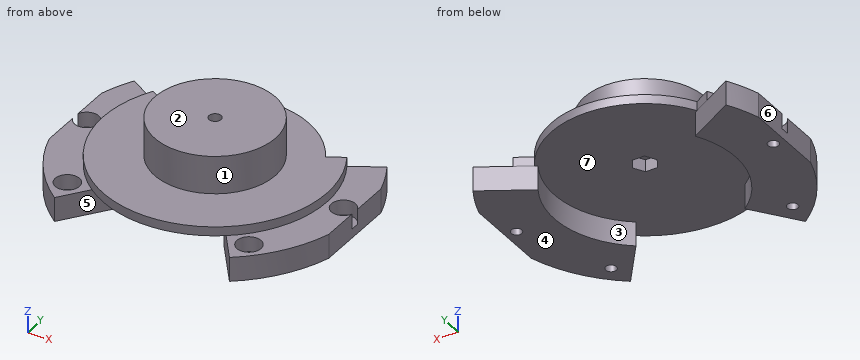
from build123d import *

# Parameters (mm, degrees)
SKETCH1_R           = 48.25
BOSS_EXTRUDE1_DEPTH = 8
SKETCH2_W           = 17.162038191
SKETCH2_H           = 56.822210482
SKETCH2_W_2         = 16.152506533
SKETCH2_H_2         = 65.186901365
CUT_EXTRUDE1_DEPTH  = 8
SKETCH3_R           = 30
CUT_EXTRUDE2_DEPTH  = 8
SKETCH4_R           = 1.75
CUT_EXTRUDE3_DEPTH  = 10
CIRPATTERN1_COUNT   = 8
CUT_EXTRUDE4_DEPTH  = 10
CIRPATTERN2_COUNT   = 2
SKETCH9_R           = 4
CUT_EXTRUDE5_DEPTH  = 5
CIRPATTERN3_COUNT   = 8
SKETCH10_R          = 4
CUT_EXTRUDE6_DEPTH  = 5
SKETCH11_R          = 37
BOSS_EXTRUDE2_DEPTH = 3
SKETCH12_R          = 20
BOSS_EXTRUDE3_DEPTH = 12.5
SKETCH13_R          = 2
CUT_EXTRUDE8_DEPTH  = 38
CUT_EXTRUDE9_DEPTH  = 4
CUT_EXTRUDE10_DEPTH = 10
CUT_EXTRUDE11_START = 14
CUT_EXTRUDE11_DEPTH = 14


with BuildPart() as part:
    # Sketch1 → Boss-Extrude1 (new body)
    with BuildSketch(Plane.XY):
        Circle(SKETCH1_R)
    extrude(amount=-BOSS_EXTRUDE1_DEPTH)

    # Sketch2 → Cut-Extrude1 (cut)
    with BuildSketch(Plane.XY):
        with Locations((-54.831019095, 0)):
            Rectangle(SKETCH2_W, SKETCH2_H)
        with Locations((54.326253267, -4.182345442)):
            Rectangle(SKETCH2_W_2, SKETCH2_H_2)
    extrude(amount=-CUT_EXTRUDE1_DEPTH, mode=Mode.SUBTRACT)

    # Sketch3 → Cut-Extrude2 (cut)
    with BuildSketch(Plane.XY):
        Circle(SKETCH3_R)
    extrude(amount=-CUT_EXTRUDE2_DEPTH, mode=Mode.SUBTRACT)

    # Sketch4 → Cut-Extrude3 (cut)
    with BuildSketch(Plane.XY):
        with Locations((-42.5, 0)):
            Circle(SKETCH4_R)
    cut_extrude3 = extrude(amount=-CUT_EXTRUDE3_DEPTH, mode=Mode.SUBTRACT)

    # CirPattern1: Cut-Extrude3 ×8 about axis
    cirpattern1_axis = Axis((0, 0, 0), (0, 0, 1))
    for i in range(1, CIRPATTERN1_COUNT):
        add(cut_extrude3.rotate(cirpattern1_axis, i * 360 / CIRPATTERN1_COUNT), mode=Mode.SUBTRACT)

    # Sketch8 → Cut-Extrude4 (cut)
    with BuildSketch(Plane.XY):
        with BuildLine():
            Line((-28.959547499, 38.59283753), (0, 0))
            Line((0, 0), (28.959547499, 38.59283753))
            ThreePointArc((28.959547499, 38.59283753), (0, 48.25), (-28.959547499, 38.59283753))
        make_face()
    cut_extrude4 = extrude(amount=-CUT_EXTRUDE4_DEPTH, mode=Mode.SUBTRACT)

    # CirPattern2: Cut-Extrude4 ×2 about axis
    cirpattern2_axis = Axis((0, 0, 0), (0, 0, 1))
    for i in range(1, CIRPATTERN2_COUNT):
        add(cut_extrude4.rotate(cirpattern2_axis, i * 360 / CIRPATTERN2_COUNT), mode=Mode.SUBTRACT)

    # Sketch9 → Cut-Extrude5 (cut)
    with BuildSketch(Plane.XY):
        with Locations((-42.5, 0)):
            Circle(SKETCH9_R)
    cut_extrude5 = extrude(amount=-CUT_EXTRUDE5_DEPTH, mode=Mode.SUBTRACT)

    # CirPattern3: Cut-Extrude5 ×8 about axis, 3 skipped
    cirpattern3_axis = Axis((0, 0, 0), (0, 0, 1))
    add([cut_extrude5.rotate(cirpattern3_axis, i * 360 / CIRPATTERN3_COUNT) for i in range(1, CIRPATTERN3_COUNT) if i not in (3, 4, 5)], mode=Mode.SUBTRACT)

    # Sketch10 → Cut-Extrude6 (cut)
    with BuildSketch(Plane.XY):
        with Locations((42.5, 0)):
            Circle(SKETCH10_R)
        with Locations((30.0520382, 30.0520382)):
            Circle(SKETCH10_R)
        with Locations((30.0520382, -30.0520382)):
            Circle(SKETCH10_R)
    extrude(amount=-CUT_EXTRUDE6_DEPTH, mode=Mode.SUBTRACT)

    # Sketch11 → Boss-Extrude2 (add)
    with BuildSketch(Plane.XY):
        with Locations(Location((0, 0, 0), (0, 0, 126.884070759))):
            Circle(SKETCH11_R)
    extrude(amount=BOSS_EXTRUDE2_DEPTH)

    # Sketch12 → Boss-Extrude3 (add)
    with BuildSketch(Plane.XY.offset(3)):
        Circle(SKETCH12_R)
    extrude(amount=BOSS_EXTRUDE3_DEPTH)

    # Sketch13 → Cut-Extrude8 (cut)
    with BuildSketch(Plane.XY.offset(15.5)):
        Circle(SKETCH13_R)
    extrude(amount=-CUT_EXTRUDE8_DEPTH, mode=Mode.SUBTRACT)

    # Sketch14 → Cut-Extrude9 (cut)
    with BuildSketch(Plane(origin=(0, 0, 0), x_dir=(-1, 0, 0), z_dir=(0, 0, -1))):
        Polygon((-2.020725942, -3.5), (2.020725942, -3.5), (4.041451884, 0), (2.020725942, 3.5), (-2.020725942, 3.5), (-4.041451884, 0), align=None)
    extrude(amount=-CUT_EXTRUDE9_DEPTH, mode=Mode.SUBTRACT)

    # Sketch15 → Cut-Extrude10 (cut)
    with BuildSketch(Plane.XY):
        with BuildLine():
            Line((-41.839011718, 24.03246967), (0, 0))
            Line((0, 0), (41.732235109, 24.217412182))
            ThreePointArc((41.732235109, 24.217412182), (-0.106776609, 48.249881852), (-41.839011718, 24.03246967))
        make_face()
    extrude(amount=-CUT_EXTRUDE10_DEPTH, mode=Mode.SUBTRACT)

    # Sketch16 → Cut-Extrude11 (cut)
    with BuildSketch(Plane.XY.offset(CUT_EXTRUDE11_START)):
        with BuildLine():
            Line((-41.839011718, 24.03246967), (-26.881023073, 15.440550462))
            ThreePointArc((-26.881023073, 15.440550462), (-0.068602588, 30.999924092), (26.812420485, 15.55937363))
            Line((26.812420485, 15.55937363), (41.732235109, 24.217412182))
            ThreePointArc((41.732235109, 24.217412182), (-0.106776609, 48.249881852), (-41.839011718, 24.03246967))
        make_face()
    extrude(amount=-CUT_EXTRUDE11_DEPTH, mode=Mode.SUBTRACT)


solid = part.part
Input: part model. Units: mm. Frame: model coordinates. Face numbers are marked on the shaded views. A direction names the side the tool comes from. Give positions to 0.01 mm unless a question says otherwise; leave off trailing zeros. Write each loop counter-clockwise with the first axis right and the second up, starting at its lowest first coordinate (ties: lowest second). Pieces come first, ordered by that corner, then holes.
Q1. First-contact query: P1, Ø10.5, axis at x = -30.05, y = -30.05, coming from the +Z side; P2, Ø8, axis at y = 19, z = 1.5, coming from the +X side; P3, Ø3, axis at x = 30.05, y = -30.05, coming from the +Z side; P4, Ø1.5, axis at x = -27, y = -2, coming from the -Z side. Flat tips, straight axial feed; report the tip coordinate or a pass-through.
Q2. Section C-C, the plane x = 21. Output: boundary loops of the cut face in (y, z), plus the area to 3 significant figures.
Q3. Section D-D, the plane x = -24.5. Output: boundary loops of the cut face in (y, z), plus the area to 3 significant figures.
Q4. Pull-direction query (X, two-part tool) for the marked faces 4, 5, 6 and 7; classes: pulls with the +X half, pulls with the -X half, needs draft (parallel to the pull), parting line crosses it, or undercut.
Q5. Set-up query: the marked faces 1, 2 and 3. Return all of +Z, -Z, +X, -X, +Y, -Y with unobstructed straight access to the full face (end or side cutting, diameter ignored); none if empty.
Q6. Material intervals for probe 1 along X at (y, z) = (0, -3.8); probe 2 along Y at (x, z) = (27, -0.5); probe 3 along Z at (x, y) = (20, 15.5), sorted ascending.
Q7. Section A-A, the plane x = 0. Output: boundary loops of the cut face in (y, z), plus the area to 3 significant figures.
Q8. Section B-B, the plane z = 6. Output: boundary loops of the cut face in (x, y), plus the area to 3 significant figures.
Filled in:
1. P1: stops at z = 0
1. P2: stops at x = 45.76
1. P3: passes through
1. P4: stops at z = 0
2. outline: (-30.46, 0) - (-27.99, 0) - (-27.99, -8) - (-21.42, -8) - (-21.42, 0) - (22.8, 0) - (22.8, 3) - (-30.46, 3) - close
2. area: 212 mm2
3. outline: (-32.65, -8) - (-17.31, -8) - (-17.31, 0) - (18.99, 0) - (18.99, 3) - (-27.73, 3) - (-27.73, 0) - (-32.65, 0) - close
3. area: 263 mm2
4. face 4: needs draft
4. face 5: undercut
4. face 6: pulls with the -X half
4. face 7: undercut
5. face 1: +Z
5. face 2: +Z, +X, -X, +Y, -Y
5. face 3: -Z
6. probe 1: x = -38.5 to -30, 30 to 38.5
6. probe 2: y = -35.98 to -32.64, -27.47 to -13.08, 13.08 to 15.67
6. probe 3: z = 0 to 3
7. outline: (-37, 0) - (-3.5, 0) - (-3.5, 4) - (-2, 4) - (-2, 15.5) - (-20, 15.5) - (-20, 3) - (-37, 3) - close; (2, 4) - (3.5, 4) - (3.5, 0) - (31, 0) - (31, 3) - (20, 3) - (20, 15.5) - (2, 15.5) - close
7. area: 630 mm2
8. outline: circle Ø40 at (0, 0); hole circle Ø4 at (0, 0)
8. area: 1,240 mm2
